```python
from build123d import *

# Parameters (mm, degrees)
SM_BASE_FLANGE_1_DEPTH = 400
CUT_EXTRUDE_1_DEPTH    = 10
FILLET_1_R             = 10
SKETCH_7_W             = 150
SKETCH_7_H             = 65
EXTRUDE_1_DEPTH        = 4
SKETCH_8_R             = 6
CUT_EXTRUDE_2_DEPTH    = 10
FILLET_2_R             = 10
FILLET_3_R             = 20
SKETCH_10_W            = 90
SKETCH_10_H            = 45
EXTRUDE_2_DEPTH        = 2
HOLE_WIZARD_7_0_7_1_D  = 7
FILLET_4_R             = 10
FILLET_5_R             = 20


# Sheet-metal steps are written as plain solids
with BuildPart() as part:
    # Sketch 1 → 基体-法兰1 (new body)
    with BuildSketch(Plane.XY):
        with BuildLine():
            Line((0, 0), (0, 67))
            ThreePointArc((0, 67), (2.343145751, 72.656854249), (8, 75))
            Line((8, 75), (90, 75))
            Line((90, 75), (90, 71))
            Line((90, 71), (8, 71))
            ThreePointArc((8, 71), (5.171572875, 69.828427125), (4, 67))
            Line((4, 67), (4, 0))
            Line((4, 0), (0, 0))
        make_face()
    extrude(amount=SM_BASE_FLANGE_1_DEPTH)

    # 草图6 → 切除-拉伸1 (cut)
    with BuildSketch(Plane.ZY):
        Polygon((0, 0), (0, 40), (70, 0), align=None)
    extrude(amount=-CUT_EXTRUDE_1_DEPTH, mode=Mode.SUBTRACT)

    # 圆角1
    fillet_1_edges = [part.edges().sort_by_distance(p)[0] for p in [
        (2, 40, 0),
        (2, 0, 70),
        (90, 73, 0),
    ]]
    fillet(fillet_1_edges, radius=FILLET_1_R)

    # 草图7 → 凸台-拉伸1 (add)
    with BuildSketch(Plane.ZY):
        with Locations((225, -32.5)):
            Rectangle(SKETCH_7_W, SKETCH_7_H)
    extrude(amount=-EXTRUDE_1_DEPTH)

    # 草图8 → 切除-拉伸2 (cut)
    with BuildSketch(Plane.ZY):
        with Locations((225, 45)):
            Circle(SKETCH_8_R)
        with BuildLine():
            Line((192.5, -35), (192.5, -13.540496218))
            ThreePointArc((192.5, -13.540496218), (185, 25), (177.5, -13.540496218))
            Line((177.5, -13.540496218), (177.5, -35))
            ThreePointArc((177.5, -35), (185, -42.5), (192.5, -35))
        make_face()
        with BuildLine():
            Line((257.5, -35), (257.5, -13.540496218))
            ThreePointArc((257.5, -13.540496218), (265, 25), (272.5, -13.540496218))
            Line((272.5, -13.540496218), (272.5, -35))
            ThreePointArc((272.5, -35), (265, -42.5), (257.5, -35))
        make_face()
    extrude(amount=-CUT_EXTRUDE_2_DEPTH, mode=Mode.SUBTRACT)

    # 圆角2
    fillet_2_edges = [part.edges().sort_by_distance(p)[0] for p in [
        (2, -13.540496218, 177.5),
        (2, -13.540496218, 192.5),
        (2, -13.540496218, 257.5),
        (2, -13.540496218, 272.5),
    ]]
    fillet(fillet_2_edges, radius=FILLET_2_R)

    # 圆角3
    fillet_3_edges = [part.edges().sort_by_distance(p)[0] for p in [
        (2, -65, 150),
        (2, 0, 150),
        (2, 0, 300),
        (2, -65, 300),
    ]]
    fillet(fillet_3_edges, radius=FILLET_3_R)

    # 草图10 → 凸台-拉伸2 (add, symmetric)
    with BuildSketch(Plane.ZY.offset(-45)):
        with Locations((60, 97.5)):
            Rectangle(SKETCH_10_W, SKETCH_10_H)
    extrude(amount=EXTRUDE_2_DEPTH, both=True)

    # Ø7.0 (7) 直径孔1 (through all)
    with Locations(Plane.ZY.offset(-43)):
        with Locations((50, 110), (70, 110)):
            Hole(HOLE_WIZARD_7_0_7_1_D / 2)

    # 圆角4
    fillet_4_edges = [part.edges().sort_by_distance(p)[0] for p in [
        (45, 120, 105),
        (45, 120, 15),
    ]]
    fillet(fillet_4_edges, radius=FILLET_4_R)

    # 圆角5
    fillet_5_edges = [part.edges().sort_by_distance(p)[0] for p in [
        (2, 0, 400),
    ]]
    fillet(fillet_5_edges, radius=FILLET_5_R)


solid = part.part
```
CAD build for the part. Positions are in the model's coordinates, mm. A direction names the side the tool comes from. Round coordinates to 2 decimals unless told otherwise and drop trailing zeros. Write each loop counter-clockwise with the first axis right and the second up, starting at its lowest first coordinate (ties: lowest second). Pieces come first, ordered by that corner, then holes. Notation, with made-up numbers: (32, 11) -> (56, 11) arc R13 cw to (56, 15) -> close; hole circle Ø6 at (-38, 26.25). An arc over 180 degrees is marked (long way). Answer in a Markdown table with one row per item. Add a question column.
Item 1: Saw through at D-D, the plane x = 76. Write the cut outline in (y, z), then the cut area to 3 significant figures.
Item 2: Saw through at B-B, the plane y = 11.5. Write the cut outline in (x, z) (3 decimals), then the cut area to 3 significant figures.
Item 3: Drop flat-ended pins along their axis: pin 1 Ø1.2 at (x, y) = (2, -38) entering from -Z; pin 2 Ø5.5 at (y, z) = (110, 70) entering from +X; pin 3 Ø1.2 at (x, y) = (45.5, 95.5) entering from +Z; pin 4 Ø24.5 at (x, z) = (58, 278) entering from +Y. Give the stop position or say it passes through.
Item 4: Mould opens along Y. For faces 1 (the face through (1.97, 19.47, 35.93)), 2 (the face through (4, 31, 197)), 3 (the face through (1.972, 24.988, 264.295)), 4 (the face through (45.028, 106.583, 70.759)) say: pulls with the +Y half, pulls with the -Y half, needs draft (parallel to the pull), parting line crosses it, or undercut.
Item 5: Which spindle directions (+Z, -Z, +X, -X, +Y, -Y) get a long thin tool onto all of the face, cutting with end or side? Do faces 5 (the face through (2.028, -5.703, 306.014)), 6 (the face through (1.97, -42.5, 184.84)), 7 (the face through (43, 98, 59)). Say none if no direction does.
Item 6: Saw through at C-C, the plane y = 82.5. Write the cut outline in (x, z), then the cut area to 3 significant figures.
Item 7: Saw through at A-A, the plane z = 265. Write the cut outline in (x, y), then the cut area to 3 significant figures.
Item 8: Drill centre lines: line 1 (Z direction, x = 1.1, y = 5); line 2 (Y direction, x = 45.15, z = 50); line 3 (Y direction, x = 27, z = 248). Where is each one in solid material? Low to high. Write a range as from..to.
Findings below:
| question | item | result |
|---|---|---|
| 1 | outline | (71, 0) -> (75, 0) -> (75, 400) -> (71, 400) -> close |
| 1 | area | 1,600 mm^2 |
| 2 | outline | (0, 49.875) -> (4, 49.875) -> (4, 166.086) -> (0, 166.086) -> close; (0, 203.914) -> (4, 203.914) -> (4, 246.086) -> (0, 246.086) -> close; (0, 283.914) -> (4, 283.914) -> (4, 398.104) -> (0, 398.104) -> close |
| 2 | area | 1,090 mm^2 |
| 3 | pin 1 | stops at z = 150 |
| 3 | pin 2 | passes through |
| 3 | pin 3 | stops at z = 105 |
| 3 | pin 4 | stops at y = 75 |
| 4 | face 1 | pulls with the -Y half |
| 4 | face 2 | needs draft |
| 4 | face 3 | undercut |
| 4 | face 4 | undercut |
| 5 | face 5 | +Z, +X, -X, -Y |
| 5 | face 6 | +X, -X |
| 5 | face 7 | +Z, -Z, -X, +Y |
| 6 | outline | (43, 15) -> (47, 15) -> (47, 105) -> (43, 105) -> close |
| 6 | area | 360 mm^2 |
| 7 | outline | (0, -65) -> (4, -65) -> (4, -42.5) -> (0, -42.5) -> close; (0, 25) -> (4, 25) -> (4, 67) arc R4 cw to (8, 71) -> (90, 71) -> (90, 75) -> (8, 75) arc R8 ccw to (0, 67) -> close |
| 7 | area | 624 mm^2 |
| 8 | line 1 | z = 61.25..165, 205..245, 285..393.23 |
| 8 | line 2 | y = 71..106.5, 113.5..120 |
| 8 | line 3 | y = 71..75 |
